Verification items for the finished model (mm, model axes). A direction names the side the tool comes from. Round coordinates to 2 decimals unless told otherwise and drop trailing zeros. Loops run counter-clockwise (first coordinate to the right, second up) from the corner with the lowest first, then second, coordinate; pieces in that order, holes last. Notation, with made-up numbers: (-17, 44.5) -> (-8, 44.5) arc R17 ccw to (-8, 49.5) -> close; hole circle Ø2 at (37.25, 7.5). An arc over 180 degrees is marked (long way). Use a Markdown table: item, result. Add a question column.
```python
from build123d import *

# Parameters (mm, degrees)
EXTRUDE_1_DEPTH     = 23
SKETCH_2_W          = 5
SKETCH_2_H          = 20
CUT_EXTRUDE_1_DEPTH = 5
CUT_EXTRUDE_2_REACH = 112.72
SKETCH_4_W          = 23
SKETCH_4_H          = 13
CUT_EXTRUDE_3_REACH = 112.72
SKETCH_3_R          = 1.5
SKETCH_7_R          = 1.5
CUT_EXTRUDE_4_DEPTH = 111.719601125
SKETCH_8_W          = 76.143558985
SKETCH_8_H          = 113.649709854
CUT_EXTRUDE_5_DEPTH = 5
SKETCH_9_W          = 28.016263666
SKETCH_9_H          = 5
SKETCH_9_W_2        = 40.160076627
CUT_EXTRUDE_6_DEPTH = 5
SKETCH_10_R         = 1.45
CUT_EXTRUDE_7_DEPTH = 114.977488026


with BuildPart() as part:
    # 草圖1 → 填料-伸長1 (new body)
    with BuildSketch(Plane.XY):
        Polygon((-17.451364004, -4.696122823), (-17.451364004, -9.696122823), (-22.451364004, -9.696122823), (-22.451364004, 100.303877177), (-17.451364004, 100.303877177), (-17.451364004, 95.303877177), (26.548635996, 95.303877177), (26.548635996, 90.303877177), (-17.451364004, 90.303877177), (-17.451364004, 0.303877177), (0.548635996, 0.303877177), (0.548635996, -4.696122823), align=None)
    extrude(amount=EXTRUDE_1_DEPTH)

    # 草圖2 → 除料-伸長1 (cut)
    with BuildSketch(Plane(origin=(0, 0, 0), x_dir=(-1, 0, 0), z_dir=(0, 0, -1))):
        with Locations((19.951364004, 42.053877177)):
            Rectangle(SKETCH_2_W, SKETCH_2_H)
    extrude(amount=-CUT_EXTRUDE_1_DEPTH, mode=Mode.SUBTRACT)

    # 草圖4 → 除料-伸長2 (cut, up to next)
    with BuildSketch(Plane(origin=(0, 95.303877177, 0), x_dir=(1, 0, 0), z_dir=(0, 1, 0)), mode=Mode.PRIVATE) as cut_extrude_2_sk1:
        with Locations((4.048635996, -6.5)):
            Rectangle(SKETCH_4_W, SKETCH_4_H)
    cut_extrude_2_tool1 = extrude(cut_extrude_2_sk1.sketch, amount=-CUT_EXTRUDE_2_REACH, mode=Mode.PRIVATE) & part.part
    add(cut_extrude_2_tool1.solids().sort_by_distance((4.048636, 95.303877, 6.5))[0], mode=Mode.SUBTRACT)

    # 草圖3 → 除料-伸長3 (cut, up to next)
    with BuildSketch(Plane.XZ.offset(4.696122823), mode=Mode.PRIVATE) as cut_extrude_3_sk1:
        with Locations((-7.451364004, 12)):
            Circle(SKETCH_3_R)
    cut_extrude_3_tool1 = extrude(cut_extrude_3_sk1.sketch, amount=-CUT_EXTRUDE_3_REACH, mode=Mode.PRIVATE) & part.part
    add(cut_extrude_3_tool1.solids().sort_by_distance((-7.451364, -4.696123, 12))[0], mode=Mode.SUBTRACT)

    # 草圖7 → 除料-伸長4 (cut, through all)
    with BuildSketch(Plane(origin=(0, 95.303877177, 0), x_dir=(1, 0, 0), z_dir=(0, 1, 0))):
        with Locations(Location((21.548635996, -12, 0), (0, 0, 270))):
            Circle(SKETCH_7_R)
    extrude(amount=-CUT_EXTRUDE_4_DEPTH, mode=Mode.SUBTRACT)

    # 草圖8 → 除料-伸長5 (cut)
    with BuildSketch(Plane(origin=(0, 0, 0), x_dir=(-1, 0, 0), z_dir=(0, 0, -1))):
        with Locations((-20.620415489, 43.47902225)):
            Rectangle(SKETCH_8_W, SKETCH_8_H)
    extrude(amount=-CUT_EXTRUDE_5_DEPTH, mode=Mode.SUBTRACT)

    # 草圖9 → 除料-伸長6 (cut)
    with BuildSketch(Plane(origin=(0, 0, 0), x_dir=(-1, 0, 0), z_dir=(0, 0, -1))):
        with Locations((31.459495837, 92.803877177)):
            Rectangle(SKETCH_9_W, SKETCH_9_H)
        with Locations((37.531402318, -2.196122823)):
            Rectangle(SKETCH_9_W_2, SKETCH_9_H)
    extrude(amount=-CUT_EXTRUDE_6_DEPTH, mode=Mode.SUBTRACT)

    # 草圖10 → 除料-伸長7 (cut, through all)
    with BuildSketch(Plane.ZY.offset(22.451364004)):
        with Locations(Location((10, 80.303877177, 0), (0, 0, 270))):
            Circle(SKETCH_10_R)
        with Locations(Location((10, 10.303877177, 0), (0, 0, 270))):
            Circle(SKETCH_10_R)
        with Locations(Location((10, 65.303877177, 0), (0, 0, 270))):
            Circle(SKETCH_10_R)
        with Locations(Location((10, 25.303877177, 0), (0, 0, 270))):
            Circle(SKETCH_10_R)
    extrude(amount=-CUT_EXTRUDE_7_DEPTH, mode=Mode.SUBTRACT)


solid = part.part
```
1) Sectioned sample at B-B on z = 2.5. Enter the section's corners in (x, y).
2) Release check for a two-part mould opening along Y. For faces 1 (the face through (-20, 0.304, 2)), 2 (the face through (-20, 100.304, 11)), 3 (the face through (26.549, 93, 14)) record: released by +Y, released by -Y, zero draft, split by the parting line, or undercut.
3) Thickness scan on line 1 (Y direction, x = -19, z = 3.5); line 2 (Y direction, x = -13, z = 12); line 3 (X direction, y = 65.5, z = 18.5). Record the ranges inside material, lowest first.
4) Go/stop test with flat-tipped pins: pin 1 (5.5 mm diameter, centred on x = -2, z = 10.5, fed in from +Y); pin 2 (4 mm diameter, centred on y = 98, z = 8, fed in from +X); pin 3 (1.5 mm diameter, centred on x = 18.5, y = 92.5, fed in from -Z). Record where each tip stops, or that it passes through.
5) Sectioned sample at C-C on z = 14.5. Enter the section's corners in (x, y).
6) Sectioned sample at D-D on y = 76.5. Enter the section's corners in (x, z), then the cut area to 3 significant figures.
7) Access from +Z, -Z, +X, -X, +Y, -Y to the whole of each face (thin tool, end or side, straight path). Record for faces 4 (the face through (-8, -4.696, 14)), 5 (the face through (-7.451, 93, 9)), 6 (the face through (-6.066, -2.231, 11.425)).
8) Sectioned sample at A-A on x = -12.5. Enter the section's corners in (y, z), then the cut area to 3 significant figures.
Geometry results:
| question | item | result |
|---|---|---|
| 1 | outline | (-22.45, -9.7) -> (-17.45, -9.7) -> (-17.45, -4.7) -> (-22.45, -4.7) -> close; (-22.45, 0.3) -> (-17.45, 0.3) -> (-17.45, 32.05) -> (-22.45, 32.05) -> close; (-22.45, 52.05) -> (-17.45, 52.05) -> (-17.45, 90.3) -> (-22.45, 90.3) -> close; (-22.45, 95.3) -> (-17.45, 95.3) -> (-17.45, 100.3) -> (-22.45, 100.3) -> close |
| 2 | face 1 | undercut |
| 2 | face 2 | released by +Y |
| 2 | face 3 | zero draft |
| 3 | line 1 | -9.7 to -4.7, 0.3 to 32.05, 52.05 to 90.3, 95.3 to 100.3 |
| 3 | line 2 | -4.7 to 0.3, 90.3 to 95.3 |
| 3 | line 3 | -22.45 to -17.45 |
| 4 | pin 1 | y = 95.3 |
| 4 | pin 2 | x = -17.45 |
| 4 | pin 3 | z = 5 |
| 5 | outline | (-22.45, -9.7) -> (-17.45, -9.7) -> (-17.45, -4.7) -> (0.55, -4.7) -> (0.55, 0.3) -> (-17.45, 0.3) -> (-17.45, 90.3) -> (26.55, 90.3) -> (26.55, 95.3) -> (-17.45, 95.3) -> (-17.45, 100.3) -> (-22.45, 100.3) -> close |
| 6 | outline | (-22.45, 0) -> (-17.45, 0) -> (-17.45, 23) -> (-22.45, 23) -> close |
| 6 | area | 115 mm^2 |
| 7 | face 4 | +Z, -Z, +X, -Y |
| 7 | face 5 | -Z, +Y |
| 7 | face 6 | -Y |
| 8 | outline | (-4.7, 5) -> (0.3, 5) -> (0.3, 23) -> (-4.7, 23) -> close; (90.3, 5) -> (95.3, 5) -> (95.3, 23) -> (90.3, 23) -> close |
| 8 | area | 180 mm^2 |
